The listing builds one solid part. Answer for the finished solid, in the listing's coordinates (mm). A direction names the side the tool comes from. Round coordinates to 2 decimals unless told otherwise and drop trailing zeros. Put each result on its own line as item: value. Start each with the question number.
```python
from build123d import *

# Parameters (mm, degrees)
SCHIZZO1_W                   = 100
SCHIZZO1_H                   = 300
ESTRUSIONE_ESTRUSIONE1_DEPTH = 15
SCHIZZO2_R                   = 2.25
TAGLIO_ESTRUSIONE1_DEPTH     = 317.583322366
SCHIZZO4_R                   = 4
TAGLIO_ESTRUSIONE2_DEPTH     = 4
SCHIZZO5_R                   = 2
TAGLIO_ESTRUSIONE3_DEPTH     = 317.583322366
FORO_PER_VITE_M4_1_D         = 4.5
FORO_PER_VITE_M4_1_DEPTH     = 10
FORO_PER_VITE_M4_1_TIP       = 1.351936393


with BuildPart() as part:
    # Schizzo1 → Estrusione-Estrusione1 (new body)
    with BuildSketch(Plane.XY):
        with Locations((50, 150)):
            Rectangle(SCHIZZO1_W, SCHIZZO1_H)
    extrude(amount=-ESTRUSIONE_ESTRUSIONE1_DEPTH)

    # Schizzo2 → Taglio-Estrusione1 (cut, through all)
    with BuildSketch(Plane.XY):
        with Locations((19.5, 105)):
            Circle(SCHIZZO2_R)
        with Locations((19.5, 5)):
            Circle(SCHIZZO2_R)
        with Locations((37, 20)):
            Circle(SCHIZZO2_R)
        with Locations((37, 46)):
            Circle(SCHIZZO2_R)
        with Locations((37, 66)):
            Circle(SCHIZZO2_R)
        with Locations((37, 92)):
            Circle(SCHIZZO2_R)
        with Locations((50, 105)):
            Circle(SCHIZZO2_R)
        with Locations((50, 5)):
            Circle(SCHIZZO2_R)
        with Locations(Location((63, 92, 0), (0, 0, 180))):
            Circle(SCHIZZO2_R)
        with Locations(Location((63, 66, 0), (0, 0, 180))):
            Circle(SCHIZZO2_R)
        with Locations(Location((63, 46, 0), (0, 0, 180))):
            Circle(SCHIZZO2_R)
        with Locations(Location((63, 20, 0), (0, 0, 180))):
            Circle(SCHIZZO2_R)
        with Locations(Location((80.5, 5, 0), (0, 0, 180))):
            Circle(SCHIZZO2_R)
        with Locations(Location((80.5, 105, 0), (0, 0, 180))):
            Circle(SCHIZZO2_R)
    extrude(amount=-TAGLIO_ESTRUSIONE1_DEPTH, mode=Mode.SUBTRACT)

    # Schizzo4 → Taglio-Estrusione2 (cut)
    with BuildSketch(Plane.XY):
        with Locations((19.5, 105)):
            Circle(SCHIZZO4_R)
        with Locations((50, 105)):
            Circle(SCHIZZO4_R)
        with Locations((80.5, 105)):
            Circle(SCHIZZO4_R)
        with Locations((37, 92)):
            Circle(SCHIZZO4_R)
        with Locations((63, 92)):
            Circle(SCHIZZO4_R)
        with Locations((37, 66)):
            Circle(SCHIZZO4_R)
        with Locations((63, 66)):
            Circle(SCHIZZO4_R)
        with Locations((37, 46)):
            Circle(SCHIZZO4_R)
        with Locations((63, 46)):
            Circle(SCHIZZO4_R)
        with Locations((19.5, 5)):
            Circle(SCHIZZO4_R)
        with Locations((37, 20)):
            Circle(SCHIZZO4_R)
        with Locations((63, 20)):
            Circle(SCHIZZO4_R)
        with Locations((50, 5)):
            Circle(SCHIZZO4_R)
        with Locations((80.5, 5)):
            Circle(SCHIZZO4_R)
    extrude(amount=-TAGLIO_ESTRUSIONE2_DEPTH, mode=Mode.SUBTRACT)

    # Schizzo5 → Taglio-Estrusione3 (cut, through all)
    with BuildSketch(Plane.XY):
        with Locations((85, 150)):
            Circle(SCHIZZO5_R)
        with Locations((85, 210)):
            Circle(SCHIZZO5_R)
        with Locations((85, 270)):
            Circle(SCHIZZO5_R)
        with Locations(Location((85, 30, 0), (0, 0, 180))):
            Circle(SCHIZZO5_R)
        with Locations(Location((85, 90, 0), (0, 0, 180))):
            Circle(SCHIZZO5_R)
        with Locations((15, 90)):
            Circle(SCHIZZO5_R)
        with Locations((15, 30)):
            Circle(SCHIZZO5_R)
        with Locations(Location((15, 270, 0), (0, 0, 180))):
            Circle(SCHIZZO5_R)
        with Locations(Location((15, 210, 0), (0, 0, 180))):
            Circle(SCHIZZO5_R)
        with Locations(Location((15, 150, 0), (0, 0, 180))):
            Circle(SCHIZZO5_R)
    extrude(amount=-TAGLIO_ESTRUSIONE3_DEPTH, mode=Mode.SUBTRACT)

    # Foro per Vite M4-1
    with Locations(Plane(origin=(15, 270, 0), x_dir=(1, 0, 0), z_dir=(0, 0, 1))):
        with Locations((0, 0), (70, 0), (0, -60), (70, -60), (0, -120), (70, -120), (0, -180), (70, -180), (0, -240), (70, -240)):
            Hole(FORO_PER_VITE_M4_1_D / 2, depth=FORO_PER_VITE_M4_1_DEPTH)
            with Locations((0, 0, -(FORO_PER_VITE_M4_1_DEPTH + FORO_PER_VITE_M4_1_TIP / 2))):  # 118° drill point
                Cone(0, FORO_PER_VITE_M4_1_D / 2, FORO_PER_VITE_M4_1_TIP, mode=Mode.SUBTRACT)


solid = part.part
```
Item 1: Determine the mould class of faces 1 (the flat face through (49, 152, 0)), 2 (the cylindrical face through (82.346, 101.451, -1.972)) for opening direction X: released by +X, released by -X, zero draft, split by the parting line, or undercut.
Item 2: A flat-ended cylindrical pin translates along its axis: pin 1 (7 mm diameter, centred on x = 50, y = 5, fed in from +Z). Find the tip coordinate at first contact, or state that the pin passes through.
Item 3: Consider line 1 along Y through (x, z) = (50, -0.85); line 2 along Y through (x, z) = (15, -4.5); line 3 along Y through (x, z) = (85.5, -14). Determine where each line is inside the solid, lowest interval first. Write a range as [from, to].
Item 4: Which of the six approach directions +Z, -Z, +X, -X, +Y, -Y give full straight-line access (tool end or side, diameter ignored) to faces 3 (the flat face through (49, 152, -15)), 4 (the cylindrical face through (21.346, 101.451, -1.972))?
Output values:
1. face 1: zero draft
1. face 2: undercut
2. pin 1: stops at z = -4
3. line 1: y = [0, 1], [9, 101], [109, 300]
3. line 2: y = [0, 27.75], [32.25, 87.75], [92.25, 147.75], [152.25, 207.75], [212.25, 267.75], [272.25, 300]
3. line 3: y = [0, 28.06], [31.94, 88.06], [91.94, 148.06], [151.94, 208.06], [211.94, 268.06], [271.94, 300]
4. face 3: -Z, +X, -X, +Y, -Y
4. face 4: +Z
